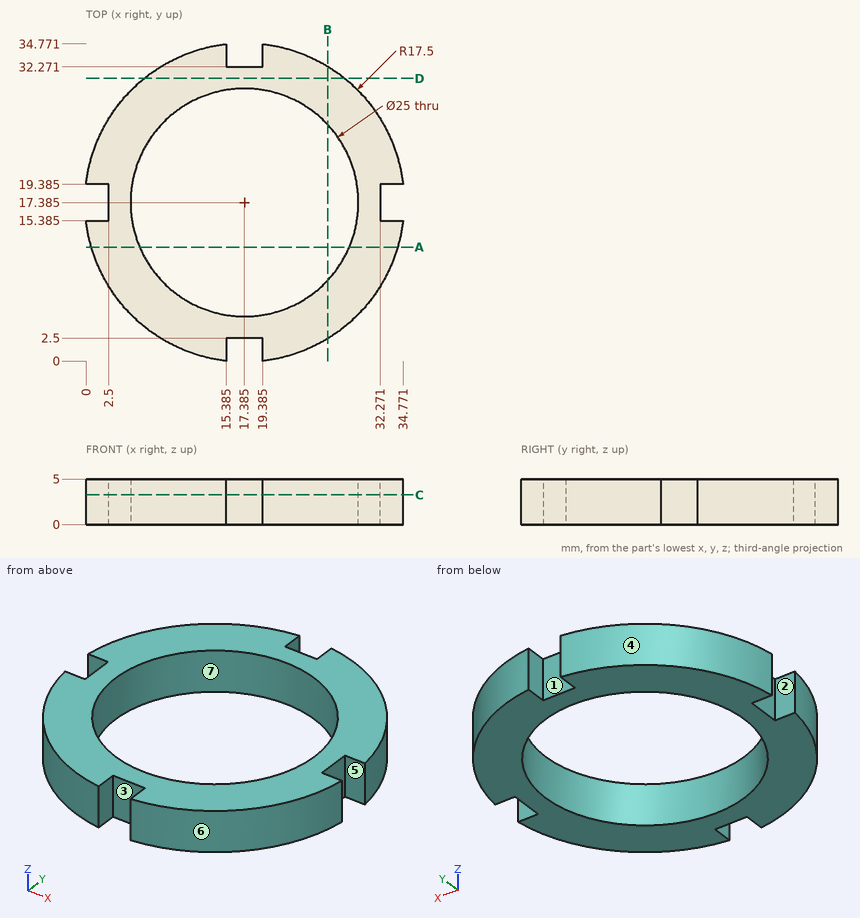
Verification items for this drawing (mm, ordinates from the low corner). A direction names the side the tool comes from. Coordinates: 2 decimals unless noted, no trailing zeros. Write each loop counter-clockwise with the first axis right and the second up, starting at its lowest first coordinate (ties: lowest second). Pieces come first, ordered by that corner, then holes. Notation, with made-up numbers: M 31.5,12.5 L 43.5,12.5 A12 cw 43.5,20.5 Z; hole C 4,77.5 d3. An arc over 180 degrees is marked long. One line per item, written item: value. Start each with the question number.
(1) Sectioned sample at D-D, the plane y = 31. Enter the section's corners in (x, z).
(2) Sectioned sample at B-B, the plane x = 26.5. Enter the section's corners in (y, z) (1 decimal).
(3) Scan lines: line 1 along X through (y, z) = (17, 2.75); line 2 along Y through (x, z) = (12, 0.55) (1 decimal); line 3 along X through (y, z) = (13, 3). Record each from-to range of solid material in increasing order. Write a range as [from, to].
(4) Depth check by flat-ended pin: pin 1 (1.2 mm diameter, centred on x = 17, z = 2, fed in from -Y); pin 2 (3 mm diameter, centred on x = 1.5, z = 3.5, fed in from +Y); pin 3 (3 mm diameter, centred on x = 10, y = 12, fed in from -Z); pin 4 (2 mm diameter, centred on x = 12, z = 1.5, fed in from -Y). Enter the tip coordinate at first touch or a pass-through.
(5) Tool access check on the marked faces 1, 2 and 3. Record the directions out of +Z, -Z, +X, -X, +Y, -Y that give a thin tool (end or side, any length) a straight path to the whole face; none if there is none.
(6) Sectioned sample at C-C, the plane z = 3.25. Enter the section's corners in (x, y) (1 decimal), and give its area (3 significant figures).
(7) Sectioned sample at A-A, the plane y = 12.5. Enter the section's corners in (x, z).
(8) Release check for a two-part mould opening along Y. For the marked faces 4, 5, 6 and 7 record: released by +Y, released by -Y, zero draft, split by the parting line, or undercut.
Filled sheet:
1. outline: M 6.39,0 L 28.38,0 L 28.38,5 L 6.39,5 Z
2. outline: M 2.4,0 L 8.8,0 L 8.8,5 L 2.4,5 Z; M 25.9,0 L 32.3,0 L 32.3,5 L 25.9,5 Z
3. line 1: [2.5, 4.89], [29.88, 32.27]
3. line 2: [0.7, 6.1], [28.7, 34]
3. line 3: [0.44, 5.68], [29.09, 34.33]
4. pin 1: y = 2.5
4. pin 2: y = 27.35
4. pin 3: through
4. pin 4: y = 0.44
5. face 1: +Z, -Z, +Y
5. face 2: +Z, -Z, -X
5. face 3: +Z, -Z, -Y
6. outline: M 0,15.4 A17.5 ccw 15.4,0 L 15.4,2.5 L 19.4,2.5 L 19.4,0 A17.5 ccw 34.8,15.4 L 32.3,15.4 L 32.3,19.4 L 34.8,19.4 A17.5 ccw 19.4,34.8 L 19.4,32.3 L 15.4,32.3 L 15.4,34.8 A17.5 ccw 0,19.4 L 2.5,19.4 L 2.5,15.4 Z; hole C 17.4,17.4 d25
6. area: 430 mm²
7. outline: M 0.58,0 L 5.88,0 L 5.88,5 L 0.58,5 Z; M 28.89,0 L 34.19,0 L 34.19,5 L 28.89,5 Z
8. face 4: released by +Y
8. face 5: undercut
8. face 6: released by -Y
8. face 7: undercut
